from build123d import *

# Parameters (mm, degrees)
F1_DEPTH = 150
F2_DEPTH = 12.5
F2_TAPER = -30


with BuildPart() as f1:
    # F0 (on Front) → F1 (new body)
    with BuildSketch(Plane.XZ):
        Polygon((6.5699621812, 11.3795083016), (-6.5699621812, 11.3795083016), (-13.1399243624, 0), (-6.5699621812, -11.3795083016), (6.5699621812, -11.3795083016), (13.1399243624, 0), align=None)
    extrude(amount=F1_DEPTH)

    # F0 (on Front) → F2 (join)
    with BuildSketch(Plane.XZ):
        Polygon((6.5699621812, 11.3795083016), (-6.5699621812, 11.3795083016), (-13.1399243624, 0), (-6.5699621812, -11.3795083016), (6.5699621812, -11.3795083016), (13.1399243624, 0), align=None)
    extrude(amount=-F2_DEPTH, taper=F2_TAPER)


solid = f1.part
Source: CAD feature listing. Evaluate the final solid. Frame: model axes, mm. A direction names the side the tool comes from. Round coordinates to 2 decimals unless told otherwise and drop trailing zeros. Loops run counter-clockwise (first coordinate to the right, second up) from the corner with the lowest first, then second, coordinate; pieces in that order, holes last. Notation, with made-up numbers: M -12,-0.5 L 17,-0.5 A31 ccw 17,35.5 Z; hole C 25,10 d4. An arc over 180 degrees is marked long. Answer as CSV lines item,"result".
Q1. Reachability of faces 1 (the face through (-9.9, -73.95, -5.61)), 2 (the face through (-9.81, -73.95, 5.77)), 3 (the face through (9.9, -73.95, 5.61)), 4 (the face through (9.81, -73.95, -5.77)), 5 (the face through (0, -74, -11.38)) from +Z, -Z, +X, -X, +Y, -Y: full face, straight path, thin tool, end or side. Return the list, or none.
Verdict:
face 1,"-Z, -X, -Y"
face 2,"+Z, -X, -Y"
face 3,"+Z, +X, -Y"
face 4,"-Z, +X, -Y"
face 5,"-Z, +X, -X, -Y"
Q2. Line query: line 1 along Z through (x, y) = (3.5, -138); line 2 along X through (y, z) = (-67, -3); line 3 along Y through (x, z) = (11, 5.5). Output: solid intervals per line, ascending.
Verdict:
line 1,"z = -11.38 to 11.38"
line 2,"x = -11.41 to 11.41"
line 3,"y = 1.55 to 12.5"
Q3. Cut plane A-A (y = -121). Return the cut outline in (x, z).
Verdict:
outline,"M -13.14,0 L -6.57,-11.38 L 6.57,-11.38 L 13.14,0 L 6.57,11.38 L -6.57,11.38 Z"
Q4. Contact query for flat-ended pins moving along their axis: pin 1 (6.5 mm diameter, centred on x = -3, y = -71.5, fed in from -Z); pin 2 (6 mm diameter, centred on x = -14, y = -22.5, fed in from +Z); pin 3 (8 mm diameter, centred on y = -15, z = -2.5, fed in from +X). Output: stop coordinate, or through.
Verdict:
pin 1,"stops at z = -11.38"
pin 2,"stops at z = 3.71"
pin 3,"stops at x = 13.14"
